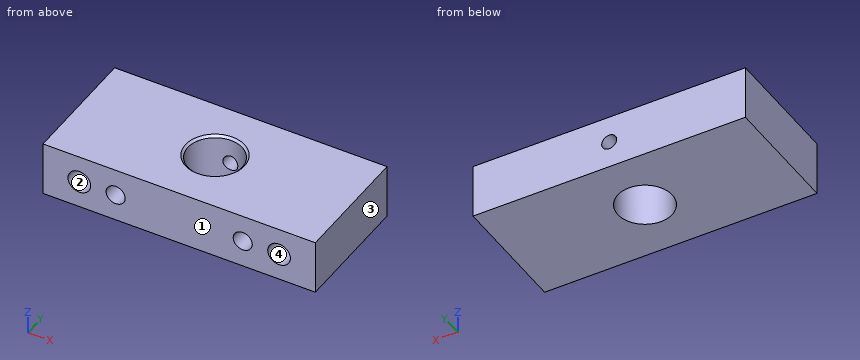
from build123d import *

# Parameters (mm, degrees)
SKETCH2_W                            = 60
SKETCH2_H                            = 27
BOSS_EXTRUDE1_DEPTH                  = 12
F_12_0MM_CLEARANCE_DOWEL_HOLE1_D     = 12
F_12_0MM_CLEARANCE_DOWEL_HOLE1_DEPTH = 12.4
F_12_0MM_CLEARANCE_DOWEL_HOLE1_TIP   = 3.605163714
M4_TAPPED_HOLE1_D                    = 3.3
M4_TAPPED_HOLE1_DEPTH                = 10.1
M4_TAPPED_HOLE1_TIP                  = 0.991420021
CHAMFER1_SIZE                        = 0.5
F_5_0MM_CLEARANCE_DOWEL_HOLE3_D      = 5
F_5_0MM_CLEARANCE_DOWEL_HOLE3_DEPTH  = 10
F_5_0MM_CLEARANCE_DOWEL_HOLE3_TIP    = 1.502151548
M5_TAPPED_HOLE3_D                    = 4.2
M5_TAPPED_HOLE3_DEPTH                = 10
M5_TAPPED_HOLE3_TIP                  = 1.2618073
M5_TAPPED_HOLE4_D                    = 4.2
M5_TAPPED_HOLE4_DEPTH                = 10
M5_TAPPED_HOLE4_TIP                  = 1.2618073
F_5_0MM_CLEARANCE_DOWEL_HOLE4_D      = 5
F_5_0MM_CLEARANCE_DOWEL_HOLE4_DEPTH  = 12.4
F_5_0MM_CLEARANCE_DOWEL_HOLE4_TIP    = 1.502151548


with BuildPart() as part:
    # Sketch2 → Boss-Extrude1 (new body)
    with BuildSketch(Plane.XY):
        with Locations((30, 13.5)):
            Rectangle(SKETCH2_W, SKETCH2_H)
    extrude(amount=BOSS_EXTRUDE1_DEPTH)

    # Ø12.0mm Clearance Dowel Hole1
    with Locations(Plane.XY.offset(12)):
        with Locations((30, 13.5)):
            Hole(F_12_0MM_CLEARANCE_DOWEL_HOLE1_D / 2, depth=F_12_0MM_CLEARANCE_DOWEL_HOLE1_DEPTH)
            with Locations((0, 0, -(F_12_0MM_CLEARANCE_DOWEL_HOLE1_DEPTH + F_12_0MM_CLEARANCE_DOWEL_HOLE1_TIP / 2))):  # 118° drill point
                Cone(0, F_12_0MM_CLEARANCE_DOWEL_HOLE1_D / 2, F_12_0MM_CLEARANCE_DOWEL_HOLE1_TIP, mode=Mode.SUBTRACT)

    # M4 Tapped Hole1
    with Locations(Plane(origin=(0, 27, 0), x_dir=(1, 0, 0), z_dir=(0, 1, 0))):
        with Locations((30, -6)):
            Hole(M4_TAPPED_HOLE1_D / 2, depth=M4_TAPPED_HOLE1_DEPTH)
            with Locations((0, 0, -(M4_TAPPED_HOLE1_DEPTH + M4_TAPPED_HOLE1_TIP / 2))):  # 118° drill point
                Cone(0, M4_TAPPED_HOLE1_D / 2, M4_TAPPED_HOLE1_TIP, mode=Mode.SUBTRACT)

    # Chamfer1
    chamfer1_edges = [part.edges().sort_by_distance(p)[0] for p in [
        (36, 13.5, 12),
    ]]
    chamfer(chamfer1_edges, length=CHAMFER1_SIZE)

    # Ø5.0mm Clearance Dowel Hole3
    with Locations(Plane(origin=(8, 0, 6), x_dir=(0, 0, -1), z_dir=(0, -1, 0))):
        with Locations((0, 0)):
            Hole(F_5_0MM_CLEARANCE_DOWEL_HOLE3_D / 2, depth=F_5_0MM_CLEARANCE_DOWEL_HOLE3_DEPTH)
            with Locations((0, 0, -(F_5_0MM_CLEARANCE_DOWEL_HOLE3_DEPTH + F_5_0MM_CLEARANCE_DOWEL_HOLE3_TIP / 2))):  # 118° drill point
                Cone(0, F_5_0MM_CLEARANCE_DOWEL_HOLE3_D / 2, F_5_0MM_CLEARANCE_DOWEL_HOLE3_TIP, mode=Mode.SUBTRACT)

    # M5 Tapped Hole3
    with Locations(Plane(origin=(16, 0, 6), x_dir=(0, 0, -1), z_dir=(0, -1, 0))):
        with Locations((0, 0)):
            Hole(M5_TAPPED_HOLE3_D / 2, depth=M5_TAPPED_HOLE3_DEPTH)
            with Locations((0, 0, -(M5_TAPPED_HOLE3_DEPTH + M5_TAPPED_HOLE3_TIP / 2))):  # 118° drill point
                Cone(0, M5_TAPPED_HOLE3_D / 2, M5_TAPPED_HOLE3_TIP, mode=Mode.SUBTRACT)

    # M5 Tapped Hole4
    with Locations(Plane(origin=(44, 0, 6), x_dir=(0, 0, -1), z_dir=(0, -1, 0))):
        with Locations((0, 0)):
            Hole(M5_TAPPED_HOLE4_D / 2, depth=M5_TAPPED_HOLE4_DEPTH)
            with Locations((0, 0, -(M5_TAPPED_HOLE4_DEPTH + M5_TAPPED_HOLE4_TIP / 2))):  # 118° drill point
                Cone(0, M5_TAPPED_HOLE4_D / 2, M5_TAPPED_HOLE4_TIP, mode=Mode.SUBTRACT)

    # Ø5.0mm Clearance Dowel Hole4
    with Locations(Plane(origin=(52, 0, 6), x_dir=(0, 0, -1), z_dir=(0, -1, 0))):
        with Locations((0, 0)):
            Hole(F_5_0MM_CLEARANCE_DOWEL_HOLE4_D / 2, depth=F_5_0MM_CLEARANCE_DOWEL_HOLE4_DEPTH)
            with Locations((0, 0, -(F_5_0MM_CLEARANCE_DOWEL_HOLE4_DEPTH + F_5_0MM_CLEARANCE_DOWEL_HOLE4_TIP / 2))):  # 118° drill point
                Cone(0, F_5_0MM_CLEARANCE_DOWEL_HOLE4_D / 2, F_5_0MM_CLEARANCE_DOWEL_HOLE4_TIP, mode=Mode.SUBTRACT)


solid = part.part
Could you check a few things on this model? Use its own coordinates, in mm. Face numbers are marked on the shaded views. Give positions to 0.01 mm unless a question says otherwise; leave off trailing zeros. Write each loop counter-clockwise with the first axis right and the second up, starting at its lowest first coordinate (ties: lowest second). Pieces come first, ordered by that corner, then holes. Notation, with made-up numbers: (-15.75, 54.5) - (8.25, 54.5) arc R32 ccw to (8.25, 80.5) - close; hole circle Ø10 at (73.5, -37). An arc over 180 degrees is marked (long way). Use CSV: the item, a comma, the result in double quotes. Start each with the question number.
Item 1: I'm going to push a flat-ended pin straight in: pin 1 (3.5 mm diameter, centred on x = 16, z = 6, fed in from -Y). Where does the tip first touch, or does it pass through?
Item 2: If I drill on line 1 along Z through (x, y) = (52, 2.5); line 2 along X through (y, z) = (24.5, 6); line 3 along X through (y, z) = (7, 6), over which ranges is the centre line in solid material (lowest first)?
Item 3: I want a section at B-B, the plane z = 1.75. Please give me the cut outline in (x, y).
Item 4: If we mould it in two halves opening along X, with no side actions, what happens to the marked faces 1, 2, 3 and 4? For each: pulls with the +X half, pulls with the -X half, needs draft (parallel to the pull), parting line crosses it, or undercut.
Item 5: I want a section at A-A, the plane y = 2.75. Please give me the cut outline in (x, z), then the cut area to 3 significant figures.
Findings:
1,pin 1,"stops at y = 10.21"
2,line 1,"z = 0 to 3.5, 8.5 to 12"
2,line 2,"x = 0 to 28.35, 31.65 to 60"
2,line 3,"x = 0 to 5.5, 10.5 to 13.9, 18.1 to 41.9, 46.1 to 49.5, 54.5 to 60"
3,outline,"(0, 0) - (60, 0) - (60, 27) - (0, 27) - close; hole circle Ø12 at (30, 13.5)"
4,face 1,"needs draft"
4,face 2,"undercut"
4,face 3,"pulls with the +X half"
4,face 4,"undercut"
5,outline,"(0, 0) - (60, 0) - (60, 12) - (0, 12) - close; hole circle Ø5 at (8, 6); hole circle Ø4.2 at (16, 6); hole circle Ø4.2 at (44, 6); hole circle Ø5 at (52, 6)"
5,area,"653 mm2"
